Verification items for the finished model (mm, model axes). Coordinates: 2 decimals unless noted, no trailing zeros. Order: outer loops, then holes, each group sorted by start corner. A loop starts at its lowest first (then second) coordinate and runs counter-clockwise, first axis right, second up. Notation, with made-up numbers: (50.5, -28.5) -> (57.5, -28.5) arc R29 cw to (57.5, 9.5) -> close; hole circle Ø2 at (50, 41). An arc over 180 degrees is marked (long way). Write each question's results on one line, items separated by ' | '. Start each with the question number.
(1) Cross-section at B-B on z = -29.78. Enter the section's corners in (x, y), and give its area (3 significant figures).
(2) Cross-section at A-A on z = 13. Enter the section's corners in (x, y) (3 decimals).
(3) Draft check along X on faces 1 (the flat face through (19, 0, 7)), 2 (the cylindrical face through (46.183, 0.74, 45.653)), 3 (the cylindrical face through (-8.514, 0.74, 45.653)). Enter one of: +X half, -X half, draft (parallel to the pull), parting line (faces both ways), or undercut.
(4) Cross-section at C-C on x = 6.5. Enter the section's corners in (y, z) (3 decimals), and give its area (3 significant figures).
(5) Cross-section at D-D on y = 0.6. Give the number of separate pieces and of enclosed holes in the cut face, and give its area (3 significant figures).
(6) Thickness scan on probe 1 along X at (y, z) = (1.1, 35) (3 decimals); probe 2 along Z at (x, y) = (27.5, 0.6) (3 decimals); probe 3 along Z at (x, y) = (5.5, 1.25) (3 decimals). Record the ranges inside material, lowest first. Write a range as [from, to].
(7) Go/stop test with flat-tipped pins: pin 1 (0.8 mm diameter, centred on x = 22.5, y = 1, fed in from -Z); pin 2 (1 mm diameter, centred on x = 1.5, z = -13, fed in from -Y); pin 3 (2 mm diameter, centred on x = -8.29, z = -29.78, fed in from +Y). Record where each tip stops, or that it passes through.
Autodesk Fusion 360 part; units mm, degrees
sketch "plate-2025-11-20T02_26_56.904Z" plane through (0, 0, 0) normal (0, 1, 0) x (1, 0, 0)
sketch "plate-2025-11-20T02_26_56.904Z (1)" plane through (0, 0, 0) normal (0, 1, 0) x (1, 0, 0)
  line L0 (3.025, -2.525) -> (16.025, -2.5274)
  line L1 (3.025, -16.525) -> (16.025, -16.525)
  line L2 (2.525, -3.025) -> (2.525, -16.025)
  line L3 (16.5157, -3.025) -> (16.5157, -16.025)
  arc A0 (3.025, -2.525) -> (2.525, -3.025) centre (3.025, -3.025) ccw
  arc A1 (16.5157, -3.025) -> (16.025, -2.5274) centre (16.0207, -3.0224) ccw
  arc A2 (2.525, -16.025) -> (3.025, -16.525) centre (3.025, -16.025) ccw
  arc A3 (16.025, -16.525) -> (16.5157, -16.025) centre (16.0194, -16.0287) ccw
  line L4 (22.105, -2.525) -> (35.105, -2.525)
  line L5 (22.105, -16.525) -> (35.105, -16.525)
  line L6 (21.5957, -3.025) -> (21.5957, -16.025)
  line L7 (35.605, -3.025) -> (35.605, -16.025)
  arc A4 (22.105, -2.525) -> (21.5957, -3.025) centre (22.1001, -3.0294) ccw
  arc A5 (35.605, -3.025) -> (35.105, -2.525) centre (35.105, -3.025) ccw
  arc A6 (21.5957, -16.025) -> (22.105, -16.525) centre (22.0993, -16.0214) ccw
  arc A7 (35.105, -16.525) -> (35.605, -16.025) centre (35.105, -16.025) ccw
  line L8 (3.025, -21.605) -> (16.025, -21.605)
  line L9 (3.025, -35.605) -> (16.025, -35.605)
  line L10 (2.525, -22.105) -> (2.525, -35.105)
  line L11 (16.525, -22.105) -> (16.525, -35.105)
  arc A8 (3.025, -21.605) -> (2.525, -22.105) centre (3.025, -22.105) ccw
  arc A9 (16.525, -22.105) -> (16.025, -21.605) centre (16.025, -22.105) ccw
  arc A10 (2.525, -35.105) -> (3.025, -35.605) centre (3.025, -35.105) ccw
  arc A11 (16.025, -35.605) -> (16.525, -35.105) centre (16.025, -35.105) ccw
  line L12 (22.105, -21.605) -> (35.105, -21.605)
  line L13 (22.105, -35.605) -> (35.105, -35.605)
  line L14 (21.605, -22.105) -> (21.605, -35.105)
  line L15 (35.605, -22.105) -> (35.605, -35.105)
  arc A12 (22.105, -21.605) -> (21.605, -22.105) centre (22.105, -22.105) ccw
  arc A13 (35.605, -22.105) -> (35.105, -21.605) centre (35.105, -22.105) ccw
  arc A14 (21.605, -35.105) -> (22.105, -35.605) centre (22.105, -35.105) ccw
  arc A15 (35.105, -35.605) -> (35.605, -35.105) centre (35.105, -35.105) ccw
  line L16 (16.5157, -12.518) -> (19.0557, -12.518)
  line L17 (19.0557, -12.518) -> (19.0557, -19)
  line L18 (19.0557, -19) -> (42.8682, -19)
  line L19 (42.8682, -19) -> (42.8682, -40.431)
  line L20 (42.8682, -40.431) -> (-4.7568, -40.431)
  line L21 (-4.7568, -40.431) -> (-4.7568, 26.244)
  line L22 (-4.7568, 26.244) -> (42.8682, 26.244)
  line L23 (42.8682, 26.244) -> (42.8682, -40.431)
  line L24 (9.8057, 26.244) -> (28.3057, 26.244)
  line L25 (-4.7568, 26.244) -> (-11.5568, 26.244)
  line L26 (-4.7568, 26.244) -> (-4.7568, 33.044)
  line L27 (42.8682, 26.244) -> (42.8682, 33.044)
  line L28 (42.8682, 26.244) -> (49.6682, 26.244)
  line L29 (42.8682, -40.431) -> (42.8682, -47.231)
  line L30 (42.8682, -40.431) -> (49.6682, -40.431)
  line L31 (-4.7568, -40.431) -> (-4.7568, -47.231)
  line L32 (-4.7568, -40.431) -> (-11.5568, -40.431)
  line L33 (-11.5568, 26.244) -> (-11.5568, 33.044)
  line L34 (42.8682, -47.231) -> (49.6682, -47.231)
  line L35 (49.6682, -47.231) -> (-11.5568, -47.231)
  line L36 (-11.5568, -47.231) -> (-11.5568, 33.044)
  line L37 (-11.5568, 33.044) -> (49.6682, 33.044)
  line L38 (49.6682, 33.044) -> (49.6682, -47.231)
  line L39 (9.8057, 26.244) -> (9.8057, 33.044)
  line L40 (9.8057, 33.044) -> (33, 33.044)
  line L41 (9.8057, 2.044) -> (9.8057, 33.044)
  line L42 (9.8057, 2.044) -> (28.3057, 2.044)
  line L43 (28.3057, 2.044) -> (9.8057, 2.044)
  line L44 (9.8057, 2.044) -> (9.8057, 33.044)
  line L45 (9.8057, 33.044) -> (28.3057, 33.044)
  line L46 (28.3057, 33.044) -> (28.3057, 2.044)
  line L47 (-4.7568, -40.431) -> (-8.2928, -40.431)
  line L48 (-8.2928, -40.431) -> (-8.2928, -43.967)
  line L49 (-4.7568, 26.244) -> (-8.2928, 26.244)
  line L50 (-8.2928, 26.244) -> (-8.2928, 29.78)
  line L51 (49.6682, 26.244) -> (46.1322, 26.244)
  line L52 (46.1322, 26.244) -> (46.1322, 29.78)
  line L53 (42.8682, -40.431) -> (46.4042, -40.431)
  line L54 (46.4042, -40.431) -> (46.4042, -43.967)
  circle A16 centre (-8.2928, -43.967) radius 1.7
  circle A17 centre (-8.2928, 29.78) radius 1.7
  circle A18 centre (46.1322, 29.78) radius 1.7
  circle A19 centre (46.4042, -43.967) radius 1.7
  point P0 (9.8057, 26.244)
  dimension "d6" = 5.08
  dimension "d7" = 5.08
  dimension "d8" = 5.08
  dimension "d9" = 5.08
  dimension "d10" = 2.54
  dimension "d12" = 23.8125
  dimension "d13" = 21.431
  dimension "d14" = 66.675
  dimension "d15" = 47.625
  dimension "d16" = 14.5625
  dimension "d18" = 21.431
  dimension "d20" = 6.8
  dimension "d21" = 6.8
  dimension "d22" = 6.8
  dimension "d23" = 6.8
  dimension "d24" = 6.8
  dimension "d25" = 6.8
  dimension "d26" = 6.8
  dimension "d27" = 6.8
  dimension "d28" = 6.8
  dimension "d29" = 6.8
  dimension "d30" = 31
  dimension "d32" = 18.5
  dimension "d33" = 3.536
  dimension "d34" = 3.536
  dimension "d35" = 3.536
  dimension "d36" = 3.536
  dimension "d37" = 3.536
  dimension "d38" = 3.536
  dimension "d39" = 3.536
  dimension "d40" = 3.536
  dimension "d41" = 3.4
  dimension "d42" = 3.4
  dimension "d43" = 3.4
  dimension "d44" = 3.4
extrude "Extrude1" add sketch "plate-2025-11-20T02_26_56.904Z (1)" along normal blind 1.5 contours L19 L20 L21 L22 L23 L41 L42 L43 L44 L46 makes body 1
extrude "Extrude2" add sketch "plate-2025-11-20T02_26_56.904Z (1)" along normal blind 1.5 separate body contours L19 L23 L28 L30 L38 L51 L53 | L29 L30 L34 L35 L38 L53 | L27 L28 L37 L38 L51 makes body 2
extrude "Extrude3" add sketch "plate-2025-11-20T02_26_56.904Z (1)" along normal blind 1.5 contours L20 L29 L31 L35 | L31 L32 L35 L36 L47 bodies 1 2
extrude "Extrude4" add sketch "plate-2025-11-20T02_26_56.904Z (1)" along normal blind 1.5 contours L21 L25 L32 L36 L47 L49 | L25 L26 L33 L36 L37 L49 bodies 1
extrude "Extrude5" add sketch "plate-2025-11-20T02_26_56.904Z (1)" along normal blind 1.5 contours L22 L26 L37 L39 L41 L44 bodies 1
extrude "Extrude6" add sketch "plate-2025-11-20T02_26_56.904Z (1)" along normal blind 1.5 contours L22 L27 L37 L40 L46 bodies 1
equation "d12 = ( 47.625 / 2 ) * 1 mm"
Results are:
1) outline: (-11.56, 0) -> (-9.99, 0) -> (-9.99, 1.5) -> (-11.56, 1.5) -> close; (-6.59, 0) -> (9.81, 0) -> (9.81, 1.5) -> (-6.59, 1.5) -> close; (28.31, 0) -> (44.43, 0) -> (44.43, 1.5) -> (28.31, 1.5) -> close; (47.83, 0) -> (49.67, 0) -> (49.67, 1.5) -> (47.83, 1.5) -> close | area: 53.9 mm2
2) outline: (-11.557, 0) -> (2.525, 0) -> (2.525, 1.5) -> (-11.557, 1.5) -> close; (16.516, 0) -> (21.596, 0) -> (21.596, 1.5) -> (16.516, 1.5) -> close; (35.605, 0) -> (49.668, 0) -> (49.668, 1.5) -> (35.605, 1.5) -> close
3) face 1: draft | face 2: undercut | face 3: undercut
4) outline: (0, -33.044) -> (1.5, -33.044) -> (1.5, 2.526) -> (0, 2.526) -> close; (0, 16.525) -> (1.5, 16.525) -> (1.5, 21.605) -> (0, 21.605) -> close; (0, 35.605) -> (1.5, 35.605) -> (1.5, 47.231) -> (0, 47.231) -> close | area: 78.4 mm2
5) separate pieces: 1 | enclosed holes: 8 | area: 3,520 mm2
6) probe 1: x = [-11.557, 2.525], [16.525, 21.605], [35.605, 49.668] | probe 2: z = [-2.044, 2.525], [16.525, 21.605], [35.605, 47.231] | probe 3: z = [-33.044, 2.525], [16.525, 21.605], [35.605, 47.231]
7) pin 1: stops at z = -2.04 | pin 2: stops at y = 0 | pin 3: passes through
